```python
from build123d import *

# Parameters (mm, degrees)
SKETCH1_W           = 25
SKETCH1_H           = 6.5
SKETCH1_W_2         = 43.15
SKETCH1_H_2         = 24.1
SKETCH1_W_3         = 14
SKETCH1_H_3         = 14
BOSS_EXTRUDE1_DEPTH = 1.5
FILLET1_R           = 3
CHAMFER1_SIZE       = 4


with BuildPart() as part:
    # Sketch1 → Boss-Extrude1 (new body)
    # profile 1 of 3: a face of its own
    with BuildSketch(Plane.XY):
        with Locations((16.525, 22.3)):
            Rectangle(SKETCH1_W, SKETCH1_H)
    # profile 2 of 3: a face of its own
    with BuildSketch(Plane.XY):
        with Locations((16.525, 7)):
            Rectangle(SKETCH1_W_2, SKETCH1_H_2)
        with Locations((26.05, 7)):
            Rectangle(SKETCH1_W_3, SKETCH1_H_3, mode=Mode.SUBTRACT)
        with Locations((7, 7)):
            Rectangle(SKETCH1_W_3, SKETCH1_H_3, mode=Mode.SUBTRACT)
    # profile 3 of 3: a face of its own
    with BuildSketch(Plane.XY):
        with Locations((16.525, -8.3)):
            Rectangle(SKETCH1_W, SKETCH1_H)
    extrude(amount=BOSS_EXTRUDE1_DEPTH)

    # Fillet1
    fillet1_edges = [part.edges().sort_by_distance(p)[0] for p in [
        (29.025, -11.55, 0.75),
        (4.025, -11.55, 0.75),
        (4.025, 25.55, 0.75),
        (29.025, 25.55, 0.75),
    ]]
    fillet(fillet1_edges, radius=FILLET1_R)

    # Chamfer1
    chamfer1_edges = [part.edges().sort_by_distance(p)[0] for p in [
        (38.1, 19.05, 0.75),
        (38.1, -5.05, 0.75),
        (-5.05, -5.05, 0.75),
        (-5.05, 19.05, 0.75),
    ]]
    chamfer(chamfer1_edges, length=CHAMFER1_SIZE)


solid = part.part
```
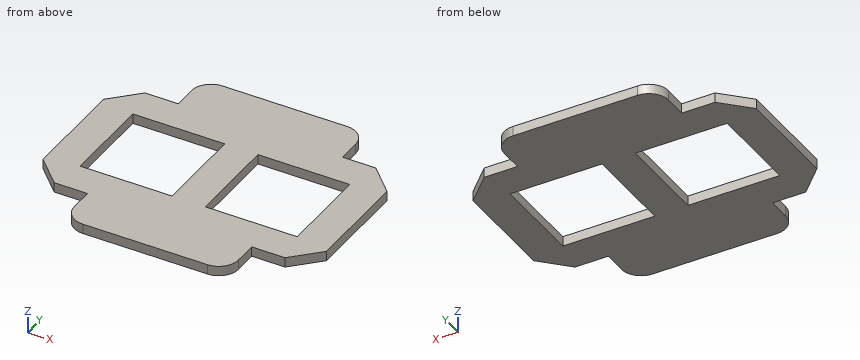
Work out the finished part from the listing and answer in its coordinate system (mm). Round coordinates to 2 decimals unless told otherwise and drop trailing zeros. Loops run counter-clockwise (first coordinate to the right, second up) from the corner with the lowest first, then second, coordinate; pieces in that order, holes last.
(1) Find the intervals of material crossed by L1, parallel to X at y = 1, z = 0.9; L2, parallel to Y at x = 32.5, z = 0.2, in increasing order.
Computed values:
L1: x = -5.05 to 0, 14 to 19.05, 33.05 to 38.1
L2: y = -5.05 to 0, 14 to 19.05
(2) The part is cut by section D-D, the plane x = 13.5. Give the vertices of the cut face in (y, z), and give its area (4 significant figures).
Computed values:
outline: (-11.55, 0) - (0, 0) - (0, 1.5) - (-11.55, 1.5) - close; (14, 0) - (25.55, 0) - (25.55, 1.5) - (14, 1.5) - close
area: 34.65 mm2
(3) Each of these flat-tipped pins is pushed along its axis until it touches: P1, Ø12, axis at x = 32.5, y = 3, coming from the -Z side; P2, Ø0.8, axis at x = 1, z = 0.5, coming from the +Y side; P3, Ø0.8, axis at y = 21.5, z = 1, coming from the -X side (3 decimals); P4, Ø0.8, axis at x = 0.5, z = 1, coming from the -Y side. Where does it stop, or does it pass through?
Computed values:
P1: stops at z = 0
P2: stops at y = 19.05
P3: stops at x = 4.025
P4: stops at y = -5.05
(4) The part is cut by section C-C, the plane y = 6. Give the vertices of the cut face in (x, z).
Computed values:
outline: (-5.05, 0) - (0, 0) - (0, 1.5) - (-5.05, 1.5) - close; (14, 0) - (19.05, 0) - (19.05, 1.5) - (14, 1.5) - close; (33.05, 0) - (38.1, 0) - (38.1, 1.5) - (33.05, 1.5) - close
(5) The part is cut by section B-B, the plane z = 0.3. Give the vertices of the cut face in (x, y) (3 decimals).
Computed values:
outline: (-5.05, -1.05) - (-1.05, -5.05) - (4.025, -5.05) - (4.025, -8.55) arc R3 ccw to (7.025, -11.55) - (26.025, -11.55) arc R3 ccw to (29.025, -8.55) - (29.025, -5.05) - (34.1, -5.05) - (38.1, -1.05) - (38.1, 15.05) - (34.1, 19.05) - (29.025, 19.05) - (29.025, 22.55) arc R3 ccw to (26.025, 25.55) - (7.025, 25.55) arc R3 ccw to (4.025, 22.55) - (4.025, 19.05) - (-1.05, 19.05) - (-5.05, 15.05) - close; hole (0, 0) - (14, 0) - (14, 14) - (0, 14) - close; hole (19.05, 0) - (33.05, 0) - (33.05, 14) - (19.05, 14) - close
(6) The part is cut by section A-A, the plane x = 3.5. Give the vertices of the cut face in (y, z), and give its area (4 significant figures).
Computed values:
outline: (-5.05, 0) - (0, 0) - (0, 1.5) - (-5.05, 1.5) - close; (14, 0) - (19.05, 0) - (19.05, 1.5) - (14, 1.5) - close
area: 15.15 mm2
